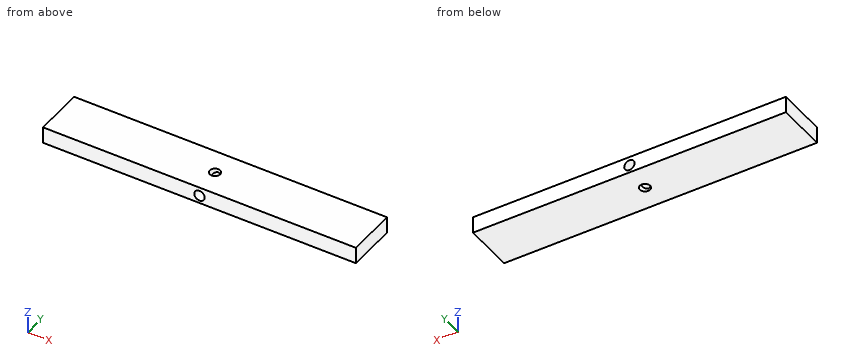
from build123d import *

# Parameters (mm, degrees)
F0_W     = 55
F0_H     = 19.05
F0_W_2   = 10
F0_R     = 2
F1_DEPTH = 6.35
F2_R     = 2
F3_DEPTH = 19.051


with BuildPart() as f1:
    # F0 (on Top) → F1 (new body)
    with BuildSketch(Plane.XY):
        with Locations((32.5, 0)):
            Rectangle(F0_W, F0_H)
        Rectangle(F0_W_2, F0_H)
        Circle(F0_R, mode=Mode.SUBTRACT)
        with Locations((-32.5, 0)):
            Rectangle(F0_W, F0_H)
    extrude(amount=F1_DEPTH)

    # F2 (on face) → F3 (cut, through all)
    with BuildSketch(Plane.XZ.offset(9.525)):
        with Locations((0, 3)):
            Circle(F2_R)
    extrude(amount=-F3_DEPTH, mode=Mode.SUBTRACT)


solid = f1.part
Source: CAD feature listing. Evaluate the final solid. Frame: model axes, mm. Round coordinates to 2 decimals unless told otherwise and drop trailing zeros. Order: outer loops, then holes, each group sorted by start corner. A loop starts at its lowest first (then second) coordinate and runs counter-clockwise, first axis right, second up. Notation, with made-up numbers: (-22.5, 45.25) -> (12.5, 45.25) arc R32 ccw to (12.5, 76.25) -> close; hole circle Ø1 at (60.5, -20). An arc over 180 degrees is marked (long way). Answer as CSV lines item,"result".
Item 1: Section A-A, the plane x = 0. Return loops of the section in (y, z) (3 decimals), plus the area to 3 significant figures.
A:
outline,"(-9.525, 0) -> (-2, 0) -> (-2, 1) -> (-9.525, 1) -> close; (-9.525, 5) -> (-2, 5) -> (-2, 6.35) -> (-9.525, 6.35) -> close; (2, 0) -> (9.525, 0) -> (9.525, 1) -> (2, 1) -> close; (2, 5) -> (9.525, 5) -> (9.525, 6.35) -> (2, 6.35) -> close"
area,"35.4 mm²"
Item 2: Pin query (flat end, axial travel): pin 1 Ø3 at (x, y) = (-15.5, -2) entering from -Z. Return the tip coordinate at first contact, or that it passes through.
A:
pin 1,"z = 0"
Item 3: Section B-B, the plane y = -4. Return loops of the section in (x, z), plus the area to 3 significant figures.
A:
outline,"(-60, 0) -> (60, 0) -> (60, 6.35) -> (-60, 6.35) -> close; hole circle Ø4 at (0, 3)"
area,"749 mm²"
Item 4: Line query: L1, parallel to X at y = -4.5, z = 2.75; L2, parallel to Y at x = 0, z = 0.95 (3 decimals); L3, parallel to Z at x = 0, y = 6. Output: solid intervals per line, ascending.
A:
L1,"-60 to -1.98, 1.98 to 60"
L2,"-9.525 to -2, 2 to 9.525"
L3,"0 to 1, 5 to 6.35"
